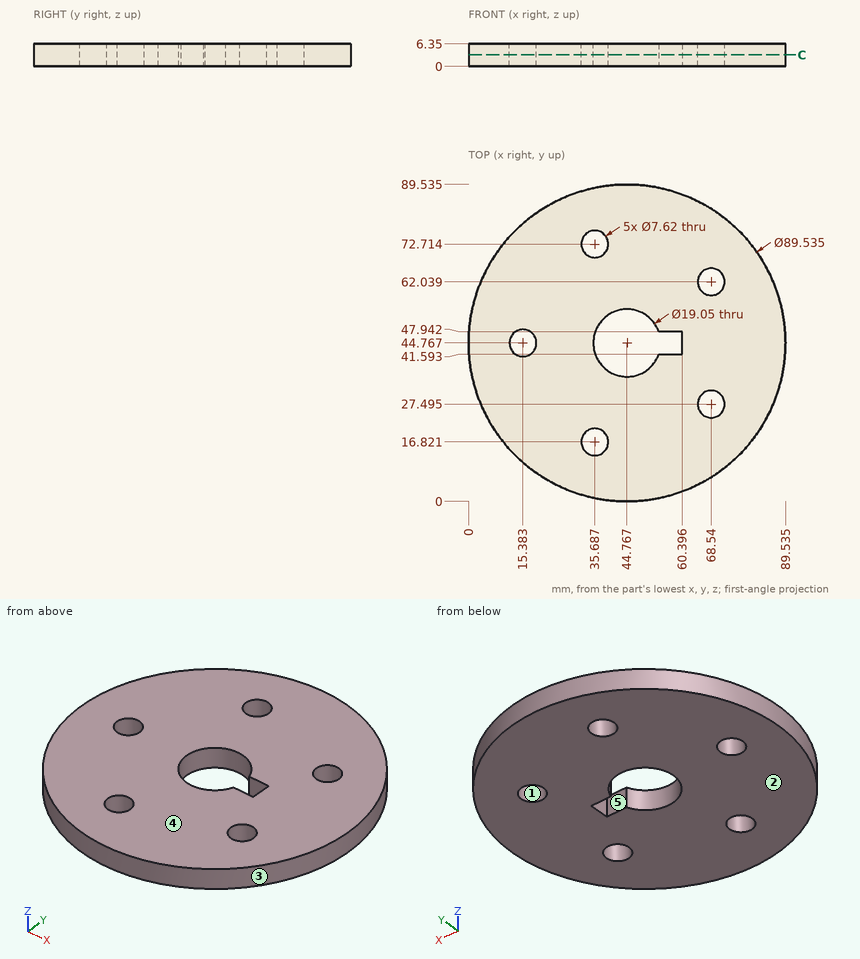
Design review of the part shown in the three views and the two pictorial views. Dimensions are in mm from the part's minimum x, y and z. A direction names the side the tool comes from. Round coordinates to 2 decimals unless told otherwise and drop trailing zeros.
Q1. Add section C-C on z = 3.25. Give the number of separate pieces and of enclosed holes in the cut face, plus the area to 3 significant figures.
Result sheet:
separate pieces: 1
enclosed holes: 6
area: 5,740 mm2
Q2. Mouldability with a two-part tool opening along X and no side actions: class the marked faces 1, 2 and 3 as +X half, -X half, draft (parallel to the pull), parting line (faces both ways), or undercut.
Result sheet:
face 1: undercut
face 2: draft
face 3: parting line
Q3. Insertion check: pin 1 Ø1 at (y, z) = (68.5, 5) entering from -X; pin 2 Ø3 at (x, z) = (57, 4.5) entering from -Y (1 decimal); pin 3 Ø3 at (x, z) = (57, 3.5) entering from +Y. Each pin has a flat end and moves straight along its axis. Give the tip position at first contact, or say it passes through.
Result sheet:
pin 1: stops at x = 6.5
pin 2: stops at y = 1.3
pin 3: stops at y = 88.23
Q4. To check wall thickness, follow line 1 along Y through (x, z) = (35, 2); line 2 along Y through (x, z) = (70.5, 3) (1 decimal); line 3 along X through (y, z) = (38.5, 5.5) (1 decimal). State the ranges of each line that lie inside material, in increasing order.
Result sheet:
line 1: y = 1.08 to 13.07, 20.57 to 68.97, 76.46 to 88.46
line 2: y = 8.1 to 24.2, 30.8 to 58.8, 65.3 to 81.4
line 3: x = 0.4 to 37.6, 51.9 to 89.1
Q5. Machinability: for the marked faces 4 and 5, which of the approach directions +Z, -Z, +X, -X, +Y, -Y give a long, thin tool a straight path to every point of the face, cutting with its end or side? Answer none if there is none.
Result sheet:
face 4: +Z, +X, -X, +Y, -Y
face 5: +Z, -Z
